Autodesk Inventor part; units mm, degrees
ref_plane "Work Plane1" through (0, 0, 17.2) normal (0, 0, 1) x (1, 0, 0)
ref_plane "Work Plane2" through (0, 0, -17.2) normal (0, 0, -1) x (-1, 0, 0)
ref_plane "YZ Plane" through (0, 0, 0) normal (1, 0, 0) x (0, 1, 0)
sketch "Sketch1" plane through (0, 0, 0) normal (0, 0, 1) x (1, 0, 0)
  circle A0 centre (0, 0) radius 1.5
  dimension "d0" = 3
extrude "Extrusion1" add sketch "Sketch1" along normal mid plane 34.4
ref_plane "Work Plane1" through (0, 0, 17.2) normal (0, 0, 1) x (1, 0, 0)
sketch "Sketch2" plane through (0, 0, 17.2) normal (0, 0, 1) x (1, 0, 0)
  circle A0 centre (0, 0) radius 2
  dimension "d4" = 4
extrude "Extrusion2" add sketch "Sketch2" along normal blind 1.5
ref_plane "Work Plane2" through (0, 0, -17.2) normal (0, 0, -1) x (-1, 0, 0)
sketch "Sketch3" plane through (0, 0, -17.2) normal (0, 0, -1) x (-1, 0, 0)
  circle A0 centre (0, 0) radius 2
extrude "Extrusion3" add sketch "Sketch3" along normal blind 1.5
fillet "Fillet1" radius 0.8 2 edges at (-2, 0, 18.7) (2, 0, -18.7)
properties part number "New_Main_Axle"
Geometry check sheet. Reference: the model listing, model coordinates, mm. Give positions to 0.01 mm unless a question says otherwise; leave off trailing zeros. Loops run counter-clockwise (first coordinate to the right, second up) from the corner with the lowest first, then second, coordinate; pieces in that order, holes last.
(1) Depth check by flat-ended pin: pin 1 Ø1 at (x, y) = (-1, 1.5) entering from -Z; pin 2 Ø2 at (x, z) = (1, -4.5) entering from -Y; pin 3 Ø2 at (y, z) = (-0.5, 5.5) entering from -X. Enter the tip coordinate at first touch or a pass-through.
From the geometry:
pin 1: stops at z = -18.69
pin 2: stops at y = -1.5
pin 3: stops at x = -1.5
(2) Thickness scan on L1, parallel to Y at x = 0.1, z = -8; L2, parallel to Z at x = -1.65, y = -0.6; L3, parallel to X at y = -0.15, z = 1. Record the ranges inside material, lowest first.
From the geometry:
L1: y = -1.5 to 1.5
L2: z = -18.48 to -17.2, 17.2 to 18.48
L3: x = -1.49 to 1.49
(3) Section check C-C on z = 0.5. Record the cut outline in (x, y), then the cut area to 3 significant figures.
From the geometry:
outline: circle Ø3 at (0, 0)
area: 7.07 mm2
(4) Section check A-A on y = 0. Record the cut outline in (x, z), then the cut area to 3 significant figures.
From the geometry:
outline: (-2, -17.9) arc R0.8 ccw to (-1.2, -18.7) - (1.2, -18.7) arc R0.8 ccw to (2, -17.9) - (2, -17.2) - (1.5, -17.2) - (1.5, 17.2) - (2, 17.2) - (2, 17.9) arc R0.8 ccw to (1.2, 18.7) - (-1.2, 18.7) arc R0.8 ccw to (-2, 17.9) - (-2, 17.2) - (-1.5, 17.2) - (-1.5, -17.2) - (-2, -17.2) - close
area: 115 mm2
(5) Release check for a two-part mould opening along Z. For faces 1 (the flat face through (0, 0, -18.7)), 2 (the cylindrical face through (-0.434, 1.952, 17.545)), 3 (the cylindrical face through (-1.5, 0.07, 0.24)) record: released by +Z, released by -Z, zero draft, split by the parting line, or undercut.
From the geometry:
face 1: released by -Z
face 2: zero draft
face 3: undercut
